Drawing for the job (mm, zero at the part's lowest x, y, z). A direction names the side the tool comes from. Give positions to 0.01 mm unless a question says otherwise; leave off trailing zeros. Loops run counter-clockwise (first coordinate to the right, second up) from the corner with the lowest first, then second, coordinate; pieces in that order, holes last. Notation, with made-up numbers: (27, 71.25) -> (81, 71.25) arc R29 cw to (81, 101.25) -> close; hole circle Ø4 at (81, 87). An arc over 180 degrees is marked (long way). Use CSV: the item, a comma, the result in double quotes. Start each with the question number.
(1) Cut at D-D on z = 6.5. Write the cut outline in (x, y), then the cut area to 3 significant figures.
(2) Cut at B-B on y = 12. Write the cut outline in (x, z).
(3) Drill centre lines: probe 1 along Y at (x, z) = (6.5, 13.8); probe 2 along X at (y, z) = (0.7, 5.5); probe 3 along Z at (x, y) = (28.5, 3.25). Where is each one in solid material? Low to high.
(4) Cut at A-A on z = 15.75. Write the cut outline in (x, y), then the cut area to 3 significant figures.
(5) Cut at C-C on x = 24. Write the cut outline in (y, z).
(6) Flat gauge pins, fed straight in: pin 1 (1 mm diameter, centred on x = 7.5, z = 9, fed in from +Y); pin 2 (4 mm diameter, centred on x = 5.5, y = 12, fed in from -Z); pin 3 (2.5 mm diameter, centred on x = 41.5, y = 12, fed in from +Z); pin 4 (2 mm diameter, centred on y = 14.5, z = 13, fed in from -X). Where does each tip first touch, or does it go through?
(7) 3-axis set-ups, long thin cutter, end or side, ignore diameter. For the marked faces 1 and 2: which of +Z, -Z, +X, -X, +Y, -Y reach the whole face in a straight line?
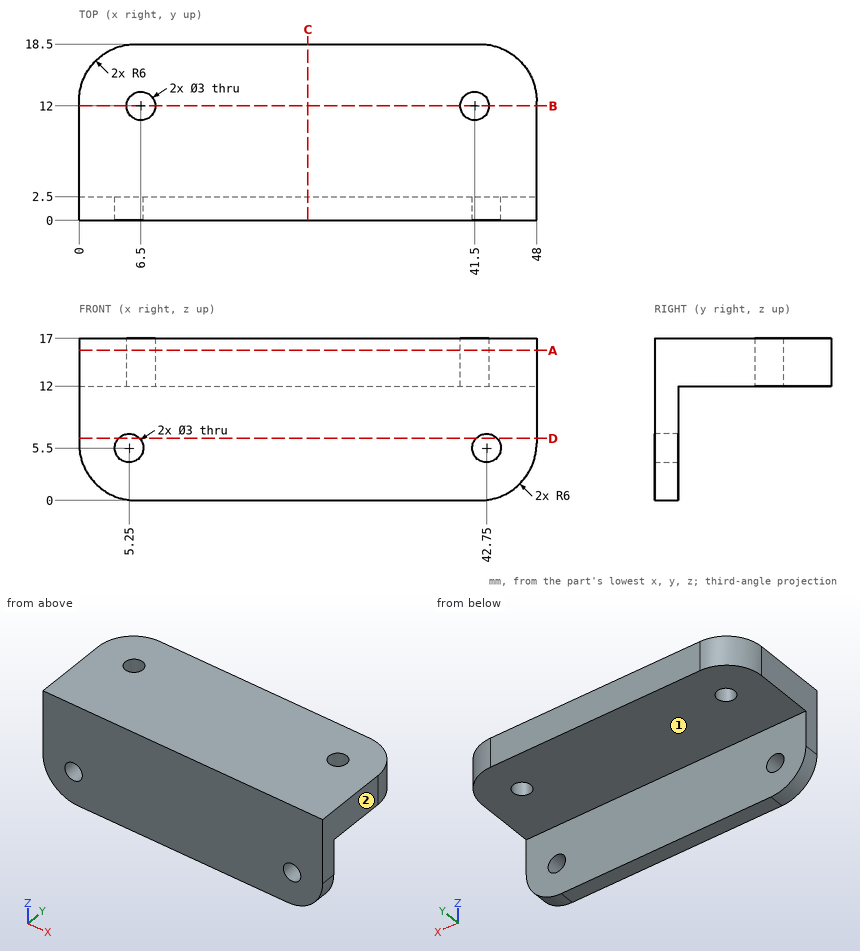
Check result:
1,outline,"(0, 0) -> (4.13, 0) -> (4.13, 2.5) -> (0, 2.5) -> close; (6.37, 0) -> (41.63, 0) -> (41.63, 2.5) -> (6.37, 2.5) -> close; (43.87, 0) -> (48, 0) -> (48, 2.5) -> (43.87, 2.5) -> close"
1,area,"109 mm²"
2,outline,"(0, 12) -> (5, 12) -> (5, 17) -> (0, 17) -> close; (8, 12) -> (40, 12) -> (40, 17) -> (8, 17) -> close; (43, 12) -> (48, 12) -> (48, 17) -> (43, 17) -> close"
3,probe 1,"0 to 10.5, 13.5 to 18.5"
3,probe 2,"0.02 to 3.75, 6.75 to 41.25, 44.25 to 47.98"
3,probe 3,"12 to 17"
4,outline,"(0, 0) -> (48, 0) -> (48, 12.5) arc R6 ccw to (42, 18.5) -> (6, 18.5) arc R6 ccw to (0, 12.5) -> close; hole circle Ø3 at (6.5, 12); hole circle Ø3 at (41.5, 12)"
4,area,"858 mm²"
5,outline,"(0, 0) -> (2.5, 0) -> (2.5, 12) -> (18.5, 12) -> (18.5, 17) -> (0, 17) -> close"
6,pin 1,"y = 2.5"
6,pin 2,"z = 12"
6,pin 3,"through"
6,pin 4,"x = 0.08"
7,face 1,"-Z, +X, -X, +Y"
7,face 2,"+Z, -Z, +X, +Y, -Y"
